Source: CAD feature listing. Evaluate the final solid. Frame: model axes, mm. A direction names the side the tool comes from. Give positions to 0.01 mm unless a question says otherwise; leave off trailing zeros. Order: outer loops, then holes, each group sorted by start corner. A loop starts at its lowest first (then second) coordinate and runs counter-clockwise, first axis right, second up. Notation, with made-up numbers: M 49.5,55.25 L 63.5,55.25 A32 ccw 63.5,86.25 Z; hole C 74.5,1.25 d11. An arc over 180 degrees is marked long. One line per question, with ' | ' between items. Start each with the question number.
from build123d import *

# Parameters (mm, degrees)
SKETCH1_R           = 21.463
BOSS_EXTRUDE1_DEPTH = 16.8
SKETCH2_R           = 1.55
BOSS_EXTRUDE2_DEPTH = 1.3
CIRPATTERN1_COUNT   = 3


with BuildPart() as part:
    # Sketch1 → Boss-Extrude1 (new body)
    with BuildSketch(Plane(origin=(0, 0, 0), x_dir=(1, 0, 0), z_dir=(0, 1, 0))):
        with Locations(Location((0, 0, 0), (0, 0, 270))):
            Circle(SKETCH1_R)
    extrude(amount=BOSS_EXTRUDE1_DEPTH)

    # Sketch2 → Boss-Extrude2 (add)
    with BuildSketch(Plane.XZ):
        with BuildLine():
            Line((-14.167399247, 16.122815126), (-16.137353009, 20.042265188))
            ThreePointArc((-16.137353009, 20.042265188), (-14.933420138, 23.679331264), (-11.296354062, 22.475398393))
            Line((-11.296354062, 22.475398393), (-9.63856212, 19.177030251))
            ThreePointArc((-9.63856212, 19.177030251), (-12.000541932, 17.794588007), (-14.167399247, 16.122815126))
        make_face()
        with Locations(Location((-13.716853536, 21.25883179, 0), (0, 0, 270))):
            Circle(SKETCH2_R, mode=Mode.SUBTRACT)
    boss_extrude2 = extrude(amount=-BOSS_EXTRUDE2_DEPTH)

    # CirPattern1: Boss-Extrude2 ×3 about axis
    cirpattern1_axis = Axis((0, 0, 0), (0, 1, 0))
    for i in range(1, CIRPATTERN1_COUNT):
        add(boss_extrude2.rotate(cirpattern1_axis, i * 360 / CIRPATTERN1_COUNT))


solid = part.part
Item 1: Pin query (flat end, axial travel): pin 1 Ø4 at (y, z) = (9.5, 18) entering from -X; pin 2 Ø2 at (x, y) = (-14.5, 3) entering from -Z; pin 3 Ø2 at (y, z) = (14, -2) entering from -X. Return the tip coordinate at first contact, or that it passes through.
Item 2: Line query: line 1 (Z direction, x = -0.5, y = 2); line 2 (Y direction, x = 26, z = -1); line 3 (X direction, y = 7.25, z = 6.5). Output: solid intervals per line, ascending.
Item 3: Cut plane A-A on y = 2. Return the cut outline in (x, z).
Item 4: Reachability of faces 1 (the flat face through (-13, 1.3, 19)), 2 (the flat face through (-12.816, 0.641, -19.5)), 3 (the flat face through (-10, 1.3, -21)) from +Z, -Z, +X, -X, +Y, -Y: full face, straight path, thin tool, end or side. Return the list, or none.
Item 5: Cut plane B-B on x = 6. Return the cut outline in (y, z), and give its area (3 significant figures).
Item 6: Cut plane C-C on z = 8.5. Return the cut outline in (x, y), and give its area (3 significant figures).
Item 7: Mould query, pull axis X, two halves, no side actions, for faces 4 (the flat face through (23.205, 0.641, 4.083)), 5 (the cylindrical face through (-13, 0.6, -24.8)), 6 (the flat face through (23, 1.3, 2)), 7 (the flat face through (23.3, 0.64, -1.35)). Classes: pulls with the +X half, pulls with the -X half, needs draft (parallel to the pull), parting line crosses it, or undercut.
Results are:
1) pin 1: stops at x = -14.31 | pin 2: stops at z = -16.69 | pin 3: stops at x = -21.44
2) line 1: z = -21.46 to 21.46 | line 2: y = 0 to 1.3 | line 3: x = -20.46 to 20.46
3) outline: C 0,0 d42.93
4) face 1: +Z, -X, +Y | face 2: -X, +Y, -Y | face 3: -Z, -X, +Y
5) outline: M 0,-20.61 L 16.8,-20.61 L 16.8,20.61 L 0,20.61 Z | area: 692 mm2
6) outline: M -19.71,0 L 19.71,0 L 19.71,16.8 L -19.71,16.8 Z | area: 662 mm2
7) face 4: pulls with the +X half | face 5: parting line crosses it | face 6: needs draft | face 7: undercut
